Model file for the job. Use its own axes, mm. Face numbers are marked on the shaded views. A direction names the side the tool comes from. Coordinates: 2 decimals unless noted, no trailing zeros. Loops run counter-clockwise (first coordinate to the right, second up) from the corner with the lowest first, then second, coordinate; pieces in that order, holes last. Notation, with made-up numbers: (33.25, 73.5) -> (70.25, 73.5) arc R21 cw to (70.25, 80.5) -> close; hole circle Ø10 at (-36.5, -7). An arc over 180 degrees is marked (long way). Use one line per item in the form item = value.
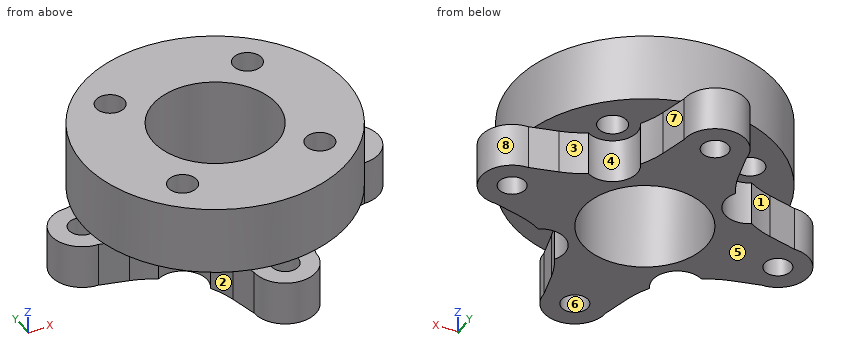
```python
from build123d import *

# Parameters (mm, degrees)
SKETCH1_R           = 1.5
SKETCH1_R_2         = 7.000334442
BOSS_EXTRUDE1_DEPTH = 5
SKETCH2_R           = 14.9
SKETCH2_R_2         = 7.000334442
BOSS_EXTRUDE2_DEPTH = 7.7
SKETCH3_R           = 1.6
CUT_EXTRUDE1_DEPTH  = 30.075574726
SKETCH4_R           = 2.8
CUT_EXTRUDE2_DEPTH  = 5


with BuildPart() as part:
    # Sketch1 → Boss-Extrude1 (new body)
    with BuildSketch(Plane.XY):
        with BuildLine():
            ThreePointArc((-6.973340003, 7.151168067), (-5.280838659, 9.337824918), (-4.251877521, 11.904392268))
            Line((-4.251877521, 11.904392268), (-3.487041473, 14.995112823))
            ThreePointArc((-3.487041473, 14.995112823), (0.012426609, 18.494580904), (3.51189469, 14.995112823))
            Line((3.51189469, 14.995112823), (4.276793265, 11.904512123))
            ThreePointArc((4.276793265, 11.904512123), (5.305826539, 9.337973695), (6.998389341, 7.151364414))
            ThreePointArc((6.998389341, 7.151364414), (7.087863136, 7.062910899), (7.176217024, 6.973338723))
            ThreePointArc((7.176217024, 6.973338723), (9.365889736, 5.275504745), (11.937407084, 4.243707607))
            Line((11.937407084, 4.243707607), (14.995112823, 3.487041473))
            ThreePointArc((14.995112823, 3.487041473), (18.494580904, -0.012426609), (14.995112823, -3.51189469))
            Line((14.995112823, -3.51189469), (11.916521074, -4.273821147))
            ThreePointArc((11.916521074, -4.273821147), (9.351558223, -5.301952454), (7.165910263, -6.992819512))
            ThreePointArc((7.165910263, -6.992819512), (7.073811789, -7.085865183), (6.980503135, -7.177697208))
            ThreePointArc((6.980503135, -7.177697208), (5.276194005, -9.371016841), (4.24095393, -11.948534758))
            Line((4.24095393, -11.948534758), (3.487041473, -14.995112823))
            ThreePointArc((3.487041473, -14.995112823), (-0.012426609, -18.494580904), (-3.51189469, -14.995112823))
            Line((-3.51189469, -14.995112823), (-4.281948892, -11.883680625))
            ThreePointArc((-4.281948892, -11.883680625), (-5.30570303, -9.326373353), (-6.988342179, -7.145406018))
            ThreePointArc((-6.988342179, -7.145406018), (-7.070989636, -7.063429863), (-7.152677278, -6.980497231))
            ThreePointArc((-7.152677278, -6.980497231), (-9.342997098, -5.281516445), (-11.915577996, -4.249109478))
            Line((-11.915577996, -4.249109478), (-14.995112823, -3.487041473))
            ThreePointArc((-14.995112823, -3.487041473), (-18.494580904, 0.012426609), (-14.995112823, 3.51189469))
            Line((-14.995112823, 3.51189469), (-11.871695344, 4.284915151))
            ThreePointArc((-11.871695344, 4.284915151), (-9.312807198, 5.30957244), (-7.130872005, 6.993909079))
            ThreePointArc((-7.130872005, 6.993909079), (-7.052543558, 7.072976887), (-6.973340003, 7.151168067))
        make_face()
        with Locations((-14.995112823, 0.012426609)):
            Circle(SKETCH1_R, mode=Mode.SUBTRACT)
        with Locations((-0.012426609, -14.995112823)):
            Circle(SKETCH1_R, mode=Mode.SUBTRACT)
        with Locations((14.995112823, -0.012426609)):
            Circle(SKETCH1_R, mode=Mode.SUBTRACT)
        with Locations((0.012426609, 14.995112823)):
            Circle(SKETCH1_R, mode=Mode.SUBTRACT)
        with Locations((0.01262523, -0.004457602)):
            Circle(SKETCH1_R_2, mode=Mode.SUBTRACT)
    extrude(amount=BOSS_EXTRUDE1_DEPTH)

    # Sketch2 → Boss-Extrude2 (add)
    with BuildSketch(Plane.XY.offset(5)):
        with Locations(Location((0.01262523, -0.004457602, 0), (0, 0, 185.670375878))):
            Circle(SKETCH2_R)
        with Locations((0.01262523, -0.004457602)):
            Circle(SKETCH2_R_2, mode=Mode.SUBTRACT)
    extrude(amount=BOSS_EXTRUDE2_DEPTH)

    # Sketch3 → Cut-Extrude1 (cut, through all)
    with BuildSketch(Plane.XY.offset(12.7)):
        with Locations((7.755444484, 7.738361652)):
            Circle(SKETCH3_R)
        with Locations((7.738361652, -7.755444484)):
            Circle(SKETCH3_R)
        with Locations((-7.755444484, -7.738361652)):
            Circle(SKETCH3_R)
        with Locations((-7.738361652, 7.755444484)):
            Circle(SKETCH3_R)
    extrude(amount=-CUT_EXTRUDE1_DEPTH, mode=Mode.SUBTRACT)

    # Sketch4 → Cut-Extrude2 (cut)
    with BuildSketch(Plane(origin=(0, 0, 0), x_dir=(-1, 0, 0), z_dir=(0, 0, -1))):
        with Locations((-7.755444484, 7.738361652)):
            Circle(SKETCH4_R)
        with Locations((7.738361652, 7.755444484)):
            Circle(SKETCH4_R)
        with Locations((7.755444484, -7.738361652)):
            Circle(SKETCH4_R)
        with Locations((-7.738361652, -7.755444484)):
            Circle(SKETCH4_R)
    extrude(amount=-CUT_EXTRUDE2_DEPTH, mode=Mode.SUBTRACT)


solid = part.part
```
Q1. Pin check, flat tips, straight feed: pin 1 Ø5 at (x, y) = (7.74, -7.76) entering from -Z; pin 2 Ø6 at (x, z) = (-4.5, 11) entering from -Y; pin 3 Ø5 at (y, z) = (-13, 10) entering from -X; pin 4 Ø2.5 at (x, y) = (-7.76, -7.74) entering from +Z. Stop position of each tip, or through.
Result:
pin_1 = 5
pin_2 = -14.83
pin_3 = -10.56
pin_4 = through
Q2. Band-saw the part on B-B, the plane z = 4.5. State how many separate pieces and enclosed holes the cut face has, and give its area (3 significant figures).
Result:
separate_pieces = 1
enclosed_holes = 5
area = 368 mm2
Q3. Band-saw the part on A-A, the plane x = -8. Write the cut outline in (y, z), and give its area (3 significant figures).
Result:
outline = (-12.57, 5) -> (-9.32, 5) -> (-9.32, 12.7) -> (-12.57, 12.7) -> close; (-6.16, 5) -> (-4.95, 5) -> (-4.95, 0) -> (4.97, 0) -> (4.97, 5) -> (6.18, 5) -> (6.18, 12.7) -> (-6.16, 12.7) -> close; (9.33, 5) -> (12.56, 5) -> (12.56, 12.7) -> (9.33, 12.7) -> close
area = 194 mm2
Q4. Band-saw the part on D-D, the plane x = 14. Write the cut outline in (y, z).
Result:
outline = (-5.14, 5) -> (-3.76, 5) -> (-3.76, 0) -> (-1.13, 0) -> (-1.13, 5) -> (1.11, 5) -> (1.11, 0) -> (3.73, 0) -> (3.73, 5) -> (5.13, 5) -> (5.13, 12.7) -> (-5.14, 12.7) -> close
Q5. Which spindle directions (+Z, -Z, +X, -X, +Y, -Y) get a long thin tool onto all of the face, cutting with end or side? Do the marked faces 1, 2, 3 and 4. Say none if no direction does.
Result:
face_1 = -Z, -X, +Y
face_2 = -Z, -X, -Y
face_3 = -Z, +X, +Y
face_4 = -Z
Q6. Band-saw the part on C-C, the plane x = -16. Write the cut outline in (y, z).
Result:
outline = (-3.34, 0) -> (-1.1, 0) -> (-1.1, 5) -> (-3.34, 5) -> close; (1.13, 0) -> (3.36, 0) -> (3.36, 5) -> (1.13, 5) -> close
Q7. Mould opens along Y. For the marked faces 5, 6, 7 and 8 say: released by +Y, released by -Y, zero draft, split by the parting line, or undercut.
Result:
face_5 = zero draft
face_6 = undercut
face_7 = released by +Y
face_8 = split by the parting line
Q8. Wall check: line 1 along Y through (x, z) = (-9, 12.25); line 2 along Z through (x, y) = (-12, -6); line 3 along X through (y, z) = (-16, 2). Give the ranges that are in metal, low to high.
Result:
line_1 = -11.87 to -8.74, -6.73 to 6.77, 8.74 to 11.86
line_2 = 5 to 12.7
line_3 = -3.36 to -1.13, 1.1 to 3.34
